```python
from build123d import *

# Parameters (mm, degrees)
HOLE_WIZARD_M561_D        = 66
HOLE_WIZARD_M561_DEPTH    = 2
SKETCH_4_R                = 25
EXTRUDE_1_DEPTH           = 2
HOLE_WIZARD_4_0_4_1_D     = 4
HOLE_WIZARD_4_0_4_1_DEPTH = 10
HOLE_WIZARD_4_0_4_2_D     = 4
HOLE_WIZARD_4_0_4_2_DEPTH = 10
CHAMFER_1_SIZE            = 1
CHAMFER_2_SIZE            = 0.5


with BuildPart() as part:
    # Эскиз1 → Повернуть1 (revolve)
    with BuildSketch(Plane.XY, mode=Mode.PRIVATE) as revolve_1_sk:
        with BuildLine():
            Line((-2, 31), (-2, 0))
            Line((-2, 0), (35, 0))
            Line((35, 0), (35, 44))
            Line((35, 44), (1, 44))
            Line((1, 44), (1, 52))
            Line((1, 52), (-5, 52))
            Line((-5, 52), (-5, 38))
            Line((-5, 38), (15.5, 38))
            ThreePointArc((15.5, 38), (19, 34.5), (15.5, 31))
            Line((15.5, 31), (-2, 31))
        make_face()
    revolve(revolve_1_sk.sketch.rotate(Axis((-5, 0, 0), (1, 0, 0)), 270), axis=Axis((-5, 0, 0), (1, 0, 0)))

    # Отверстие с зазором M561
    with Locations(Plane(origin=(35, 0, 0), x_dir=(0, 0, -1), z_dir=(1, 0, 0))):
        with Locations((0, 0)):
            Hole(HOLE_WIZARD_M561_D / 2, depth=HOLE_WIZARD_M561_DEPTH)

    # Эскиз4 → Бобышка-Вытянуть1 (add)
    with BuildSketch(Plane(origin=(33, 0, 0), x_dir=(0, 0, -1), z_dir=(1, 0, 0))):
        with Locations(Location((0, 0, 0), (0, 0, 180))):
            Circle(SKETCH_4_R)
    extrude(amount=EXTRUDE_1_DEPTH)

    # Эскиз5 → Вырез-Повернуть1 (revolve, cut)
    with BuildSketch(Plane.XY, mode=Mode.PRIVATE) as cut_revolve_1_sk:
        Polygon((-2, 29), (-2, 0), (35, 0), (35, 21), (5, 21), (5, 18), (0, 18), (0, 29), align=None)
    revolve(cut_revolve_1_sk.sketch.rotate(Axis((-2, 0, 0), (1, 0, 0)), 270), axis=Axis((-2, 0, 0), (1, 0, 0)), mode=Mode.SUBTRACT)

    # Диаметр отверстия Ø4.0 (4)1
    with Locations(Plane(origin=(35, 0, 0), x_dir=(0, 0, -1), z_dir=(1, 0, 0))):
        with Locations((-32.908965344, -19), (0, 38), (32.908965344, 19), (32.908965344, -19), (0, -38), (-32.908965344, 19)):
            Hole(HOLE_WIZARD_4_0_4_1_D / 2, depth=HOLE_WIZARD_4_0_4_1_DEPTH)

    # Диаметр отверстия Ø4.0 (4)2
    with Locations(Plane.ZY):
        with Locations((20.784609691, 12), (-20.784609691, 12), (0, -24), (20.784609691, -12), (-20.784609691, -12), (0, 24)):
            Hole(HOLE_WIZARD_4_0_4_2_D / 2, depth=HOLE_WIZARD_4_0_4_2_DEPTH)

    # Фаска1
    chamfer_1_edges = [part.edges().sort_by_distance(p)[0] for p in [
        (35, 0, 21),
    ]]
    chamfer(chamfer_1_edges, length=CHAMFER_1_SIZE)

    # Фаска2
    chamfer_2_edges = [part.edges().sort_by_distance(p)[0] for p in [
        (35, 19, 30.908965344),
        (35, -38, -2),
        (35, -19, -34.908965344),
        (35, 19, -34.908965344),
        (35, 38, -2),
        (35, -19, 30.908965344),
        (0, 24, 2),
        (0, -12, -18.784609691),
        (0, -12, 22.784609691),
        (0, -24, 2),
        (0, 12, -18.784609691),
        (0, 12, 22.784609691),
    ]]
    chamfer(chamfer_2_edges, length=CHAMFER_2_SIZE)


solid = part.part
```
Work out the finished part from the listing and answer in its coordinate system (mm). A direction names the side the tool comes from. Give positions to 0.01 mm unless a question says otherwise; leave off trailing zeros. Order: outer loops, then holes, each group sorted by start corner. A loop starts at its lowest first (then second) coordinate and runs counter-clockwise, first axis right, second up. Notation, with made-up numbers: (-5.5, 83) - (34.5, 83) arc R20 ccw to (34.5, 99) - close; hole circle Ø5 at (-24.75, -23). An arc over 180 degrees is marked (long way). One line per item, written item: value. Start each with the question number.
1. Consider line 1 (Y direction, x = 2.4, z = 0); line 2 (Y direction, x = 18.5, z = 11.5); line 3 (Y direction, x = 33.5, z = 16). Determine where each line is inside the solid, lowest interval first.
2. Which of the six approach directions +Z, -Z, +X, -X, +Y, -Y give full straight-line access (tool end or side, diameter ignored) to faces 1 (the face through (10, -24, 0)), 2 (the face through (34, -12.6, 30.5)), 3 (the face through (2.465, 5.407, -17.169))?
3. Each of these flat-tipped pins is pushed along its axis until it touches: pin 1 Ø4.5 at (y, z) = (-12, -20.78) entering from -X; pin 2 Ø4.5 at (y, z) = (24, -0.5) entering from -X; pin 3 Ø12 at (x, z) = (22, 16) entering from +Y. Where does it stop, or does it pass through?
4. Section B-B, the plane x = 31.5 is taken. Write down the section's boundary in (y, z).
5. Section A-A, the plane x = 13 is taken. Write down the section's boundary in (y, z), then the cut area to 3 significant figures.
6. For a pull along Y with two mould halves and no side action, classify faces 4 (the face through (-2.042, -31.641, 41.265)), 5 (the face through (25, -19, -33)) as released by +Y, released by -Y, zero draft, split by the parting line, or undercut.
Filled sheet:
1. line 1: -44 to -38, -31 to -26, -22 to -18, 18 to 22, 26 to 31, 38 to 44
1. line 2: -42.47 to -34.43, -30.61 to -17.57, 17.57 to 30.61, 34.43 to 42.47
1. line 3: -40.99 to -28.86, -19.21 to -13.6, 13.6 to 19.21, 28.86 to 40.99
2. face 1: -X
2. face 2: +X
2. face 3: +X, -X
3. pin 1: x = 0.25
3. pin 2: x = 0
3. pin 3: y = 42.85
4. outline: circle Ø88 at (0, 0); hole circle Ø4 at (-38, 0); hole circle Ø4 at (-19, -32.91); hole circle Ø42 at (0, 0); hole circle Ø4 at (-19, 32.91); hole circle Ø4 at (19, -32.91); hole circle Ø4 at (19, 32.91); hole circle Ø4 at (38, 0)
5. outline: circle Ø88 at (0, 0); circle Ø62 at (0, 0); hole circle Ø76 at (0, 0); hole circle Ø42 at (0, 0)
5. area: 3,180 mm²
6. face 4: split by the parting line
6. face 5: undercut
